Read the model definition and answer for the solid it produces. Units are mm, in the model's axes. A direction names the side the tool comes from. Give positions to 0.01 mm unless a question says otherwise; leave off trailing zeros. Loops run counter-clockwise (first coordinate to the right, second up) from the corner with the lowest first, then second, coordinate; pieces in that order, holes last.
(1) Find section D-D, the plane z = 34. State how many separate pieces and enclosed holes the cut face has, then the cut area to 3 significant figures.
(2) Each of these flat-tipped pins is pushed along its axis until it touches: P1, Ø3, axis at x = -15.5, z = 17.5, coming from the +Y side; P2, Ø1.5, axis at x = 14, z = -35, coming from the +Y side; P3, Ø3, axis at x = 4, z = -27, coming from the +Y side. Where does it stop, or does it pass through?
(3) Straight lines are drawn through the part: probe 1 along X at (y, z) = (14, -31); probe 2 along Y at (x, z) = (-4.5, 45); probe 3 along Y at (x, z) = (0.5, 15). For each, find the intervals that lie inside material, in ascending order.
(4) Determine the mould class of faces 1 (the face through (-16.27, 0.72, -39.86)), 2 (the face through (-0.273, 17.082, -37.254)), 3 (the face through (22.111, 20.566, 0.7)), 4 (the face through (0, -11, 30)) for opening direction X: pulls with the +X half, pulls with the -X half, needs draft (parallel to the pull), parting line crosses it, or undercut.
(5) Which of the six approach directions +Z, -Z, +X, -X, +Y, -Y give full straight-line access (tool end or side, diameter ignored) to faces 5 (the face through (-21.32, 21.34, 0.7)), 6 (the face through (-2, -40, 0)), 7 (the face through (11.91, -54.96, 0.7))?
(6) Find section C-C, the plane x = -6. Write down the section's boundary in (y, z), then the cut area to 3 significant figures.
(7) Find section B-B, the plane y = 15. Write down the section's boundary in (x, z), then the cut area to 3 significant figures.
```python
from build123d import *

# Parameters (mm, degrees)
BOSS_EXTRUDE1_DEPTH     = 50
FILLET1_R               = 12.5
FILLET2_R               = 40
CUT_EXTRUDE1_DEPTH      = 80.72452587
CUT_EXTRUDE1_DEPTH_BACK = 80.72452587
SKETCH7_W               = 60
SKETCH7_H               = 40
FILLET3_R               = 10
BOSS_EXTRUDE2_DEPTH     = 50
FILLET5_R               = 40
CUT_EXTRUDE2_DEPTH      = 83.117686393
CUT_EXTRUDE2_DEPTH_BACK = 83.117686393
SKETCH9_W               = 60
SKETCH9_H               = 18
FILLET4_R               = 10
CUT_EXTRUDE3_DEPTH      = 120.345357801
CUT_EXTRUDE3_DEPTH_BACK = 120.345357801
SKETCH10_R              = 2.1


with BuildPart() as part:
    # Sketch4 → Boss-Extrude1 (new, symmetric)
    with BuildSketch(Plane.XY):
        with BuildLine():
            ThreePointArc((8, 0), (0, -8), (-8, 0))
            Line((-8, 0), (-16, 0))
            ThreePointArc((-16, 0), (-15.099668871, -5.291502622), (-12.5, -9.987492178))
            Line((-12.5, -9.987492178), (-12.5, -58.683472972))
            ThreePointArc((-12.5, -58.683472972), (-6.284569266, -59.669960526), (0, -60))
            ThreePointArc((0, -60), (6.682717176, -59.945089422), (13.363629715, -59.780372517))
            Line((13.363629715, -59.780372517), (10.416666667, -50))
            ThreePointArc((10.416666667, -50), (8.869060232, -29.858930271), (12.5, -9.987492178))
            ThreePointArc((12.5, -9.987492178), (15.099668871, -5.291502622), (16, 0))
            Line((16, 0), (8, 0))
        make_face()
    extrude(amount=BOSS_EXTRUDE1_DEPTH, both=True)

    # Fillet1
    fillet1_edges = [part.edges().sort_by_distance(p)[0] for p in [
        (-12.5, -58.683472972, 0),
    ]]
    fillet(fillet1_edges, radius=FILLET1_R - 0.0001)  # a hair under: the kernel refuses the full size

    # Fillet2
    fillet2_edges = [part.edges().sort_by_distance(p)[0] for p in [
        (-12.5, -9.987492178, 0),
        (12.5, -9.987492178, 0),
    ]]
    fillet(fillet2_edges, radius=FILLET2_R)

    # Sketch7 → Cut-Extrude1 (cut, two sides: drawn at the far end of the back side and taken through both)
    with BuildSketch(Plane(origin=(0, 0, 0), x_dir=(0, 0, -1), z_dir=(1, 0, 0)).offset(-CUT_EXTRUDE1_DEPTH_BACK)):
        with Locations((0, -20)):
            Rectangle(SKETCH7_W, SKETCH7_H)
    extrude(amount=CUT_EXTRUDE1_DEPTH + CUT_EXTRUDE1_DEPTH_BACK, mode=Mode.SUBTRACT)

    # Fillet3
    fillet3_edges = [part.edges().sort_by_distance(p)[0] for p in [
        (-1.752259827, -40, -30),
        (-1.752259827, -40, 30),
    ]]
    fillet(fillet3_edges, radius=FILLET3_R)

    # Sketch8 → Boss-Extrude2 (add, symmetric)
    with BuildSketch(Plane.XY):
        with BuildLine():
            Line((8, 0), (16, 0))
            ThreePointArc((16, 0), (0, 16), (-16, 0))
            Line((-16, 0), (-8, 0))
            ThreePointArc((-8, 0), (0, 8), (8, 0))
        make_face()
        with BuildLine():
            ThreePointArc((-16, 0), (0, 16), (16, 0))
            Line((16, 0), (16, 37.1510767))
            ThreePointArc((16, 37.1510767), (-4.673406093, 40.179121139), (-24.099890471, 32.486886266))
            Line((-24.099890471, 32.486886266), (-16, 0))
        make_face()
        with BuildLine():
            Line((16, 37.1510767), (16, 0))
            Line((16, 0), (25.363643105, 31.510127078))
            ThreePointArc((25.363643105, 31.510127078), (20.873256116, 34.648371955), (16, 37.1510767))
        make_face()
    extrude(amount=BOSS_EXTRUDE2_DEPTH, both=True)

    # Fillet5
    fillet5_edges = [part.edges().sort_by_distance(p)[0] for p in [
        (-16, 0, 40),
        (16, 0, 40),
        (-16, 0, -40),
        (16, 0, -40),
    ]]
    fillet(fillet5_edges, radius=FILLET5_R)

    # Sketch9 → Cut-Extrude2 (cut, two sides: drawn at the far end of the back side and taken through both)
    with BuildSketch(Plane(origin=(0, 0, 0), x_dir=(0, 0, -1), z_dir=(1, 0, 0)).offset(-CUT_EXTRUDE2_DEPTH_BACK)):
        with Locations((0, 9)):
            Rectangle(SKETCH9_W, SKETCH9_H)
    extrude(amount=CUT_EXTRUDE2_DEPTH + CUT_EXTRUDE2_DEPTH_BACK, mode=Mode.SUBTRACT)

    # Fillet4
    fillet4_edges = [part.edges().sort_by_distance(p)[0] for p in [
        (0.430514749, 18, 30),
        (0.430514749, 18, -30),
    ]]
    fillet(fillet4_edges, radius=FILLET4_R - 0.0001)  # a hair under: the kernel refuses the full size

    # Sketch10 → Cut-Extrude3 (cut, two sides: drawn at the far end of the back side and taken through both)
    with BuildSketch(Plane.XY.offset(50).offset(-CUT_EXTRUDE3_DEPTH_BACK)):
        with Locations((0, 15)):
            Circle(SKETCH10_R)
        with Locations((0, -15)):
            Circle(SKETCH10_R)
    extrude(amount=CUT_EXTRUDE3_DEPTH + CUT_EXTRUDE3_DEPTH_BACK, mode=Mode.SUBTRACT)


solid = part.part
```
Entries:
1. separate pieces: 1
1. enclosed holes: 3
1. area: 2,760 mm2
2. P1: stops at y = 37.95
2. P2: stops at y = 38.22
2. P3: stops at y = 40.37
3. probe 1: x = -19.49 to -1.85, 1.85 to 20.16
3. probe 2: y = -59.16 to -6.61, 6.61 to 40.2
3. probe 3: y = -60 to -40, 18 to 40.45
4. face 1: pulls with the -X half
4. face 2: undercut
4. face 3: pulls with the +X half
4. face 4: needs draft
5. face 5: +Z, -Z, -X, -Y
5. face 6: +X, -X
5. face 7: +Z, -Z, +X
6. outline: (-58.47, -50) - (-5.29, -50) - (-5.29, -30) - (-30, -30) arc R10 cw to (-40, -20) - (-40, 20) arc R10 cw to (-30, 30) - (-5.29, 30) - (-5.29, 50) - (-58.47, 50) - close; (5.29, -50) - (40, -50) - (40, 50) - (5.29, 50) - (5.29, 30) - (8, 30) arc R10 cw to (18, 20) - (18, -20) arc R10 cw to (8, -30) - (5.29, -30) - close
6. area: 6,030 mm2
7. outline: (-19.74, -50) - (-2.1, -50) - (-2.1, -27.14) - (-19.74, -27.14) - close; (-19.74, 27.14) - (-2.1, 27.14) - (-2.1, 50) - (-19.74, 50) - close; (2.1, -50) - (20.46, -50) - (20.46, -27.14) - (2.1, -27.14) - close; (2.1, 27.14) - (20.46, 27.14) - (20.46, 50) - (2.1, 50) - close
7. area: 1,650 mm2
